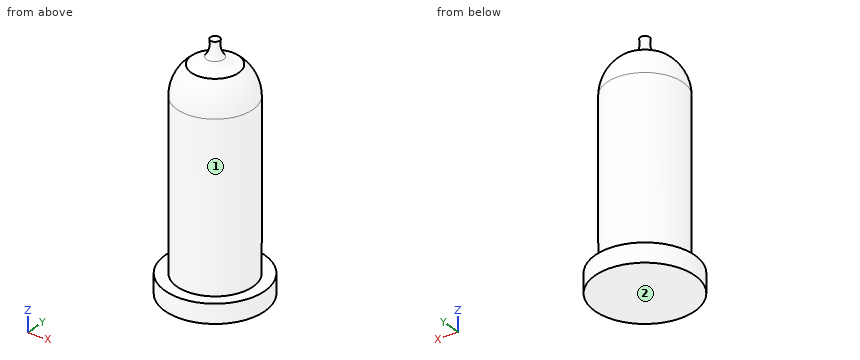
from build123d import *

# Parameters (mm, degrees)
F0_R     = 10.5
F1_DEPTH = 4
F2_R     = 8
F3_DEPTH = 39


with BuildPart() as f1:
    # F0 (on Top) → F1 (new body)
    with BuildSketch(Plane.XY):
        Circle(F0_R)
    extrude(amount=F1_DEPTH)

    # F2 (on Top) → F3 (join)
    with BuildSketch(Plane.XY):
        Circle(F2_R)
    extrude(amount=F3_DEPTH)

    # F4 (on Right) → F5 (revolve)
    with BuildSketch(Plane.YZ):
        with BuildLine():
            Line((5, 45.244998), (0, 45.244998))
            Line((0, 45.244998), (0, 39))
            Line((0, 39), (8, 39))
            ThreePointArc((8, 39), (7.211103, 42.464102), (5, 45.244998))
        make_face()
        with BuildLine():
            Line((0, 50.244998), (0, 47))
            ThreePointArc((0, 47), (0.899322, 46.949291), (1.787243, 46.797805))
            ThreePointArc((1.787243, 46.797805), (1.002907, 48.432173), (1, 50.244998))
            Line((1, 50.244998), (0, 50.244998))
        make_face()
        with BuildLine():
            ThreePointArc((1.787243, 46.797805), (0.899322, 46.949291), (0, 47))
            Line((0, 47), (0, 45.244998))
            Line((0, 45.244998), (5, 45.244998))
            ThreePointArc((5, 45.244998), (3.215832, 45.653556), (1.787243, 46.797805))
        make_face()
    revolve(axis=Axis((0, 0, 43), (0, 0, -1)))


solid = f1.part
For this review, take the finished solid that the model builds, in its own axes (mm). Face numbers are marked on the shaded views. A direction names the side the tool comes from. Give positions to 0.01 mm unless a question says otherwise; leave off trailing zeros. Order: outer loops, then holes, each group sorted by start corner. A loop starts at its lowest first (then second) coordinate and runs counter-clockwise, first axis right, second up. Notation, with made-up numbers: M 60.5,71 L 81.5,71 A21 cw 81.5,85 Z; hole C 48,69.5 d9. An arc over 180 degrees is marked long. Answer in a Markdown table with one row per item. Add a question column.
(1) For the marked faces 1 and 2, list the 3-axis set-ups (+Z, -Z, +X, -X, +Y, -Y) from which the entire face can be reached by the end or side of a thin tool; tool diameter is ignored.
(2) For pin 1 (12 mm diameter, centred on x = 4, y = 8, fed in from +Z); pin 2 (5 mm diameter, centred on x = 3.5, z = 12.5, fed in from +Y); pin 3 (3 mm diameter, centred on y = -0.5, z = 8, fed in from -X), all flat-tipped, find the tip position at first contact; note any pin that passes through.
(3) Wall thickness on probe 1 along Z at (x, y) = (-3, 8.5); probe 2 along Z at (x, y) = (-0.25, 5); probe 3 along Y at (x, z) = (-6.25, 11.5): over which ranges is each line inside the solid? List them lowest first. Write a range as [from, to].
(4) Consider section A-A on z = 34. State the section outline as (x, y) points.
(5) Consider section B-B on x = 8.5. State the section outline as (y, z) points.
Evaluation:
| question | item | result |
|---|---|---|
| 1 | face 1 | +Z |
| 1 | face 2 | -Z, +X, -X, +Y, -Y |
| 2 | pin 1 | stops at z = 45.8 |
| 2 | pin 2 | stops at y = 7.94 |
| 2 | pin 3 | stops at x = -8 |
| 3 | probe 1 | z = [0, 4] |
| 3 | probe 2 | z = [0, 45.24] |
| 3 | probe 3 | y = [-4.99, 4.99] |
| 4 | outline | C 0,0 d16 |
| 5 | outline | M -6.16,0 L 6.16,0 L 6.16,4 L -6.16,4 Z |
